Read the model definition and answer for the solid it produces. Units are mm, in the model's axes. Face numbers are marked on the shaded views. A direction names the side the tool comes from. Coordinates: 2 decimals unless noted, no trailing zeros. Order: outer loops, then holes, each group sorted by start corner. A loop starts at its lowest first (then second) coordinate and runs counter-clockwise, first axis right, second up. Notation, with made-up numbers: M 54.25,25.25 L 70.25,25.25 A18 cw 70.25,36.25 Z; hole C 86,-7 d7. An arc over 180 degrees is marked long. Write each question's results on one line, items separated by ' | '.
Autodesk Inventor part; units mm, degrees
ref_plane "YZ Plane" through (0, 0, 0) normal (1, 0, 0) x (0, 1, 0)
ref_plane "XZ Plane" through (0, 0, 0) normal (0, 1, 0) x (-1, 0, 0)
ref_plane "XY Plane" through (0, 0, 0) normal (0, 0, 1) x (1, 0, 0)
ref_plane "Work Plane1" through (0, 0, 0) normal (0, 0, 1) x (1, 0, 0)
sketch "Sketch1" plane through (0, 0, 0) normal (0, 0, 1) x (1, 0, 0)
  circle A0 centre (0, 0) radius 25.9979
  circle A1 centre (-9.4998, -11.0022) radius 2.6601
  circle A2 centre (0.0001, -0.0022) radius 3.8801
  circle A3 centre (0.0001, -0.0022) radius 6.7754
  circle A4 centre (0.0001, -0.0022) radius 10
  point P0 (0, 0)
  dimension "d17" = 20
extrude "Extrusion1" add sketch "Sketch1" along normal blind 10 contours A0 | A1 | A2 | A3 | A4
ref_plane "Arbeitsebene4" through (0, 0, 5) normal (0, 0, -1) x (-1, 0, 0)
sketch "Skizze22" plane through (0, 0, 10) normal (0, 0, 1) x (1, 0, 0)
  circle A0 centre (0, 0) radius 25.9979
  line L0 (-9.5, 60.9958) -> (9.5, 60.9958)
  line L1 (9.5, 60.9958) -> (9.5, -9)
  line L2 (9.5, -9) -> (-9.5, -9)
  line L3 (-9.5, -9) -> (-9.5, 60.9958)
  line L4 (-9.5, 60.9958) -> (9.5, -9) construction
  line L5 (9.5, 60.9958) -> (-9.5, -9) construction
  point P0 (0, 0)
  point P1 (0, 25.9979)
  point P2 (2.05, -9)
  dimension "d82" = 19
extrude "Extrusion16" cut sketch "Skizze22" against normal blind 10 contours L1 L2 L3 A0 | A0 L3 L0 L1 picked at (-1.0778, 2.5987)
sketch "Skizze23" plane through (0, 0, 5) normal (0, 0, -1) x (-1, 0, 0)
  line L0 (-5.5015, 4.1) -> (-5.3008, 4.7)
  line L1 (-5.3008, 4.7) -> (5.3257, 4.7)
  line L2 (5.3257, 4.7) -> (5.5015, 4.1)
  line L3 (5.5015, 4.1) -> (5.65, 3.9515)
  line L4 (5.65, 3.9515) -> (5.65, -4)
  line L5 (4.85, -4) -> (5.65, -4)
  arc A0 (4.05, -3.2) -> (4.85, -4) centre (4.85, -3.2) ccw
  line L6 (4.05, -3.2) -> (4.05, 1.7)
  line L7 (4.05, 1.7) -> (2.85, 1.7)
  line L8 (2.85, -3.2) -> (2.85, 1.7)
  arc A1 (2.05, -4) -> (2.85, -3.2) centre (2.05, -3.2) ccw
  line L9 (-2.05, -4) -> (2.05, -4)
  arc A2 (-2.85, -3.2) -> (-2.05, -4) centre (-2.05, -3.2) ccw
  line L10 (-2.85, -3.2) -> (-2.85, 1.7)
  line L11 (-2.85, 1.7) -> (-4.05, 1.7)
  line L12 (-4.05, -3.2) -> (-4.05, 1.7)
  arc A3 (-4.85, -4) -> (-4.05, -3.2) centre (-4.85, -3.2) ccw
  line L13 (-5.65, -4) -> (-4.85, -4)
  line L14 (-5.65, -4) -> (-5.65, 3.9515)
  line L15 (-5.65, 3.9515) -> (-5.5015, 4.1)
  line L16 (5.65, -4) -> (5.65, -7)
  line L17 (5.65, -7) -> (7.5, -7)
  line L18 (7.5, -7) -> (7.5, -9)
  line L19 (7.5, -9) -> (4.85, -9)
  line L20 (4.85, -6) -> (4.85, -9)
  line L21 (4.85, -4) -> (4.85, -6)
  line L22 (4.85, -4) -> (5.65, -4)
  line L23 (-5.65, -7) -> (-5.65, -4)
  line L24 (-5.65, -4) -> (-4.85, -4)
  line L25 (-4.85, -4) -> (-4.85, -6)
  line L26 (-4.85, -6) -> (-4.85, -9)
  line L27 (-4.85, -9) -> (-7.5, -9)
  line L28 (-7.5, -9) -> (-7.5, -7)
  line L29 (-7.5, -7) -> (-5.65, -7)
  line L30 (-4.85, -9) -> (4.85, -9)
  line L31 (5.65, -7) -> (5.3257, -7)
  line L32 (5.3257, -7) -> (5.3257, 4.7)
  line L33 (5.3257, 4.7) -> (5.65, 4.7)
  line L34 (5.65, 4.7) -> (5.65, -7)
  line L35 (-5.3008, 4.7) -> (-5.65, 4.7)
  line L36 (-5.65, 4.7) -> (-5.65, -7)
  line L37 (-5.65, -7) -> (-5.3008, -7)
  line L38 (-5.3008, -7) -> (-5.3008, 4.7)
  point P0 (5.3257, -4)
  point P1 (-5.3008, -4)
extrude "Extrusion17" add sketch "Skizze23" along normal mid plane 1.7 contours L1 L32 L5 A0 L6 L7 L8 A1 L9 A2 L10 L11 L12 A3 L13 L38 | L38 L37 L23 L13 | L13 L25 L26 L27 L28 L29 L37 L38 | L32 L31 L17 L18 L19 L20 L21 L5 | L5 L16 L31 L32 | A3 L12 L11 L10 A2 L9 A1 L8 L7 L6 A0 L21 L20 L30 L26 L25
sketch "Skizze24" plane through (0, 0, 5.85) normal (0, 0, -1) x (1, 0, 0)
  line L0 (2.85, 3.2) -> (2.85, -1.7)
  line L1 (2.85, -1.7) -> (4.05, -1.7)
  line L2 (4.05, 3.2) -> (4.05, -1.7)
  arc A0 (4.85, 4) -> (4.05, 3.2) centre (4.85, 3.2) ccw
  line L3 (4.85, 4) -> (4.85, 6)
  arc A1 (2.85, 3.2) -> (2.05, 4) centre (2.05, 3.2) ccw
  line L4 (2.05, 4) -> (2.05, 6)
  line L5 (4.85, 6) -> (4.85, 9)
  line L6 (2.05, 6) -> (2.05, 9)
  line L7 (9.5, 9) -> (-9.5, 9)
  line L8 (-2.05, 6) -> (-2.05, 9)
  line L9 (-4.85, 6) -> (-4.85, 9)
  line L10 (-2.15, 5.5641) -> (-2.15, 4)
  line L11 (-2.05, 4) -> (-2.05, 6)
  line L12 (-4.85, 4) -> (-4.85, 6)
  arc A2 (-4.05, 3.2) -> (-4.85, 4) centre (-4.85, 3.2) ccw
  arc A3 (-2.05, 4) -> (-2.85, 3.2) centre (-2.05, 3.2) ccw
  line L13 (-2.85, 3.2) -> (-2.85, -1.7)
  line L14 (-4.05, 3.2) -> (-4.05, -1.7)
  line L15 (-4.05, -1.7) -> (-2.85, -1.7)
extrude "Extrusion18" cut sketch "Skizze24" along normal blind 1
sketch "Skizze25" plane through (-9.5, -9, 10) normal (0, 1, 0) x (1, 0, 0)
  line L0 (14.4863, 5) -> (11.4863, 5)
  line L1 (11.4863, 5) -> (11.4863, 2)
  line L2 (11.4863, 2) -> (14.4863, 2)
  line L3 (14.4863, 2) -> (14.4863, 5)
  line L4 (7.4938, 5) -> (4.4938, 5)
  line L5 (4.4938, 5) -> (4.4938, 2)
  line L6 (4.4938, 2) -> (7.4938, 2)
  line L7 (7.4938, 2) -> (7.4938, 5)
  line L8 (19, 0) -> (0, 0)
  line L9 (19, 0) -> (19, 10)
  line L10 (0, 10) -> (19, 10)
  line L11 (0, 0) -> (0, 10)
  point P0 (9.5, 10)
  dimension "d90" = 3
  dimension "d91" = 3
  dimension "d92" = 3
  dimension "d93" = 3
extrude "Extrusion19" cut sketch "Skizze25" against normal through all contours L3 L2 L1 L0 | L7 L6 L5 L4
sketch "Skizze26" plane through (0, 0, 10) normal (0, 0, 1) x (1, 0, 0)
  line L0 (9.5, 24.2) -> (9.5, -9)
  line L1 (9.5, -9) -> (-9.5, -9)
  line L2 (-9.5, -9) -> (-9.5, 24.2)
  arc A0 (-9.5, 24.2) -> (9.5, 24.2) centre (0, 0) ccw
  line L3 (-14, 14.1304) -> (14, 14.1304) construction
  line L4 (-14, 10.6304) -> (14, 10.6304)
  line L5 (14, 17.6304) -> (-14, 17.6304)
  arc A1 (-14, 17.6304) -> (-14, 10.6304) centre (-14, 14.1304) ccw
  arc A2 (14, 10.6304) -> (14, 17.6304) centre (14, 14.1304) ccw
  point P0 (0, 0)
  point P1 (0, 14.1304)
  dimension "d96" = 14
  dimension "d97" = 7
extrude "Extrusion20" cut sketch "Skizze26" against normal blind 4 contours L5 A2 L4 L0 | L0 L4 L2 L5 | L2 L4 A1 L5
sketch "Skizze27" plane through (0, 0, 0) normal (0, 0, -1) x (-1, 0, 0)
  line L0 (-9.5, 10.6304) -> (-9.5, 17.6304)
  line L1 (-14, 10.6304) -> (-9.5, 10.6304)
  arc A0 (-14, 17.6304) -> (-14, 10.6304) centre (-14, 14.1304) ccw
  line L2 (-9.5, 17.6304) -> (-14, 17.6304)
  line L3 (9.5, 17.6304) -> (9.5, 10.6304)
  line L4 (14, 17.6304) -> (9.5, 17.6304)
  arc A1 (14, 10.6304) -> (14, 17.6304) centre (14, 14.1304) ccw
  line L5 (9.5, 10.6304) -> (14, 10.6304)
  line L6 (9.5, 17.6304) -> (9.5, 10.6304)
  line L7 (-9.5, 17.6304) -> (-14, 17.6304)
  line L8 (9.5, 10.6304) -> (-9.5, 10.6304)
  line L9 (-9.5, 10.6304) -> (-9.5, 17.6304)
  line L10 (-9.5, 17.6304) -> (9.5, 17.6304)
  line L11 (9.5, 17.6304) -> (9.5, 10.6304)
  point P0 (0, 0)
extrude "Extrusion21" add sketch "Skizze27" against normal blind 3
sketch "Skizze28" plane through (0, 0, 0) normal (0, 0, -1) x (-1, 0, 0)
  arc A0 (-14, 17.6304) -> (-14, 10.6304) centre (-14, 14.1304) ccw
  arc A1 (14, 10.6304) -> (14, 17.6304) centre (14, 14.1304) ccw
  circle A2 centre (-14, 14.1304) radius 1.4
  circle A3 centre (14, 14.1304) radius 1.4
  point P0 (0, 0)
  dimension "d102" = 2.8
  dimension "d103" = 2.8
extrude "Extrusion22" cut sketch "Skizze28" against normal through all
fillet "Rundung3" radius 2 2 edges at (9.5, 24.2, 5) (-9.5, 24.2, 5)
ref_plane "Arbeitsebene5" through (0, 0, 5) normal (0, 0, 1) x (1, 0, 0)
sketch "Skizze29" plane through (0, 0, 10) normal (0, 0, 1) x (1, 0, 0)
  point P0 (0, 0)
sketch "Skizze30" plane through (0, 0, 10) normal (0, 0, 1) x (1, 0, 0)
  circle A0 centre (-17.4978, -9.9998) radius 1.3999
  circle A1 centre (-17.4979, 10.0001) radius 1.4
  circle A2 centre (17.5021, 10.0001) radius 1.4
  circle A3 centre (17.5021, -9.9999) radius 1.4001
  circle A4 centre (0.0022, 0.0001) radius 3.95
  circle A5 centre (11.0022, -9.4998) radius 2.6601
  line L0 (19.0307, -17.7122) -> (18.4312, -14.7304)
  line L1 (18.4312, -14.7304) -> (15.4222, -13.716)
  line L2 (15.4222, -13.716) -> (13.0391, -15.8146)
  line L3 (13.0391, -15.8146) -> (13.6651, -18.9277)
  line L4 (13.6651, -18.9277) -> (16.6741, -19.9422)
  line L5 (16.6741, -19.9422) -> (17.7641, -18.9823)
  arc A6 (7.7254, -24.8235) -> (17.7641, -18.9823) centre (0, 0) ccw
  arc A7 (6.496, -23.8502) -> (7.7254, -24.8235) centre (7.496, -23.8502) ccw
  line L6 (6.496, -23.8502) -> (6.496, -17.7002)
  arc A8 (6.496, -17.7002) -> (4.496, -15.7002) centre (4.496, -17.7002) ccw
  line L7 (4.496, -15.7002) -> (-3.4917, -15.7002)
  arc A9 (-3.4917, -15.7002) -> (-5.4917, -17.7002) centre (-3.4917, -17.7002) ccw
  line L8 (-5.4917, -17.7002) -> (-5.4917, -24.1417)
  arc A10 (-6.6998, -25.1198) -> (-5.4917, -24.1417) centre (-6.4917, -24.1417) ccw
  arc A11 (-25.545, 4.8315) -> (-6.6998, -25.1198) centre (0, 0) ccw
  line L9 (-25.545, 4.8315) -> (-24.0265, 3.1166)
  line L10 (-24.0265, 3.1166) -> (-20.9151, 3.751)
  line L11 (-20.9151, 3.751) -> (-19.9088, 6.7628)
  line L12 (-19.9088, 6.7628) -> (-22.0139, 9.1401)
  line L13 (-22.0139, 9.1401) -> (-24.5243, 8.6283)
  arc A12 (-9.6986, 24.1211) -> (-24.5243, 8.6283) centre (0, 0) ccw
  line L14 (-9.6986, 24.1211) -> (-10.2078, 21.7325)
  line L15 (-10.2078, 21.7325) -> (-7.8493, 19.6063)
  line L16 (-7.8493, 19.6063) -> (-4.8287, 20.5857)
  line L17 (-4.8287, 20.5857) -> (-4.1666, 23.6914)
  line L18 (-4.1666, 23.6914) -> (-5.9577, 25.306)
  arc A13 (19.0307, -17.7122) -> (-5.9577, 25.306) centre (0, 0) ccw
  point P0 (0, 0)
hole "Bohrung2" at (-17.4978, -9.9998, 10) at (-17.4979, 10.0001, 10) at (17.5021, -9.9999, 10) at (17.5021, 10.0001, 10) direction (0, 0, -1) diameter 2.9 depth 7 tip angle 118
ref_plane "Arbeitsebene6" through (0, -9, 0) normal (-1, 0, 0) x (0, 0, 1)
sketch "Skizze32" plane through (-9.5, 17.6304, 0) normal (0, 1, 0) x (1, 0, 0)
  line L0 (14.8008, -5.85) -> (14.8008, -4.15)
  line L1 (4.1743, -4.15) -> (14.8008, -4.15)
  line L2 (4.1743, -5.85) -> (4.1743, -4.15)
  line L3 (14.8008, -5.85) -> (4.1743, -5.85)
  line L4 (16.8008, -2.15) -> (16.8008, -7.85)
  line L5 (16.8008, -7.85) -> (2.1743, -7.85)
  line L6 (2.1743, -7.85) -> (2.1743, -2.15)
  line L7 (2.1743, -2.15) -> (16.8008, -2.15)
  point P0 (9.5, 0)
  dimension "d116" = 2
extrude "Extrusion24" cut sketch "Skizze32" against normal blind 7 contours L3 L2 L1 L0 | L4 L5 L6 L7
properties part number "Matchboxscope_layer_ikealamp"
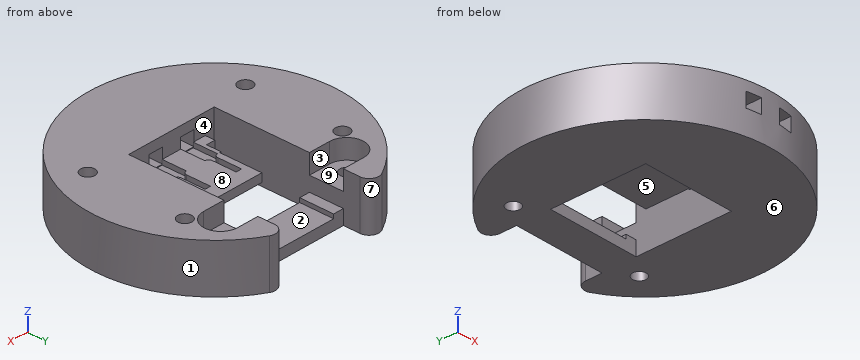
(1) The part is cut by section A-A, the plane y = 0. Write down the section's boundary in (x, z), then the cut area to 3 significant figures.
Conclusion:
outline: M -26,0 L -9.5,0 L -9.5,10 L -26,10 Z; M -5.33,4.15 L 5.3,4.15 L 5.3,5.85 L 4.05,5.85 L 4.05,4.85 L 2.85,4.85 L 2.85,5.85 L -2.85,5.85 L -2.85,4.85 L -4.05,4.85 L -4.05,5.85 L -5.33,5.85 Z; M 9.5,0 L 26,0 L 26,10 L 9.5,10 Z | area: 346 mm²
(2) The mould has two halves that part along Y. Classify the marked faces 1, 2, 3 and 4: pulls with the +Y half, pulls with the -Y half, needs draft (parallel to the pull), parting line crosses it, or undercut.
Conclusion:
face 1: parting line crosses it | face 2: needs draft | face 3: undercut | face 4: undercut
(3) The part is cut by section C-C, the plane y = -16.5. Write down the section's boundary in (x, z), then the cut area to 3 significant figures.
Conclusion:
outline: M -20.09,0 L 20.09,0 L 20.09,10 L -20.09,10 Z; hole M -5.01,5 L -2.01,5 L -2.01,8 L -5.01,8 Z; hole M 1.99,5 L 4.99,5 L 4.99,8 L 1.99,8 Z | area: 384 mm²
(4) Straight lines are drawn through the part: line 1 (X direction, y = 13, z = 4.5); line 2 (X direction, y = -10.5, z = 9.5); line 3 (Y direction, x = -0.5, z = 1). For each, find the intervals that lie inside material, in ascending order.
Conclusion:
line 1: -22.51 to -14.83, -13.17 to -9.5, 9.5 to 13.17, 14.83 to 22.51 | line 2: -23.78 to -18.86, -16.14 to 16.14, 18.86 to 23.78 | line 3: -25.99 to -9, 10.63 to 17.63
(5) For the marked faces 5, 6, 7, 8 and 9, determine the directions among +Z, -Z, +X, -X, +Y, -Y from which every point of the face is accessible in a straight line to the end or side of a thin tool.
Conclusion:
face 5: -Z, +Y | face 6: -Z, +X, -X, +Y, -Y | face 7: +Z, -Z, +Y | face 8: +Z, +Y | face 9: +Z
(6) The part is cut by section B-B, the plane x = 0. Write down the section's boundary in (y, z).
Conclusion:
outline: M -26,0 L -9,0 L -9,4.15 L 4.7,4.15 L 4.7,5.85 L -9,5.85 L -9,10 L -26,10 Z; M 10.63,0 L 17.63,0 L 17.63,2.15 L 10.63,2.15 Z
(7) Given pin 1 (7 mm diameter, centred on x = 3, y = 0.5, fed in from -Z); pin 2 (0.5 mm diameter, centred on y = -0.5, z = 5.5, fed in from -X); pin 3 (1.5 mm diameter, centred on x = -2.5, y = 11, fed in from +Z); pin 4 (2 mm diameter, centred on x = -12, y = -6, fed in from -Z), each flat-ended and moving along its own axis, determine where each tip first touches the part or whether it passes through.
Conclusion:
pin 1: z = 4.15 | pin 2: x = -26 | pin 3: z = 2.15 | pin 4: z = 0
(8) The part is cut by section D-D, the plane x = -10.5. Write down the section's boundary in (y, z).
Conclusion:
outline: M -23.78,0 L 22.8,0 L 22.8,10 L 17.63,10 L 17.63,6 L 10.63,6 L 10.63,10 L -23.78,10 Z
